The drawing under review shows one solid part. Ordinate dimensions are in mm from its lowest x, y, z. A direction names the side the tool comes from. Coordinates: 2 decimals unless noted, no trailing zeros. Write each loop counter-clockwise with the first axis right and the second up, starting at its lowest first coordinate (ties: lowest second). Pieces come first, ordered by that corner, then holes.
1) Add section D-D, the plane y = 47. State the section outline as (x, z) points.
2) Add section B-B, the plane x = 8. State the section outline as (y, z) points.
3) Mouldability with a two-part tool opening along X and no side actions: class the marked faces 1, 2 and 3 as released by +X, released by -X, zero draft, split by the parting line, or undercut.
4) Add section C-C, the plane z = 4.5. State the section outline as (x, y) points.
5) Machinability: for the marked faces 4, 5 and 6, which of the approach directions +Z, -Z, +X, -X, +Y, -Y give a long, thin tool a straight path to every point of the face, cutting with its end or side? Answer none if there is none.
6) For P1, Ø2, axis at x = 14, z = 3.5, coming from the +Y side; P2, Ø6, axis at x = 20.5, y = 10, coming from the +Z side, all flat-tipped, find the tip position at first contact; note any pin that passes through.
7) Add section A-A, the plane y = 26. State the section outline as (x, z) points.
8) For line 1 (X direction, y = 29, z = 3.5); line 2 (Y direction, x = 8.5, z = 3.5); line 3 (Z direction, x = 21, y = 47.5), list the stretches that pass through material, from the lowest coordinate up.
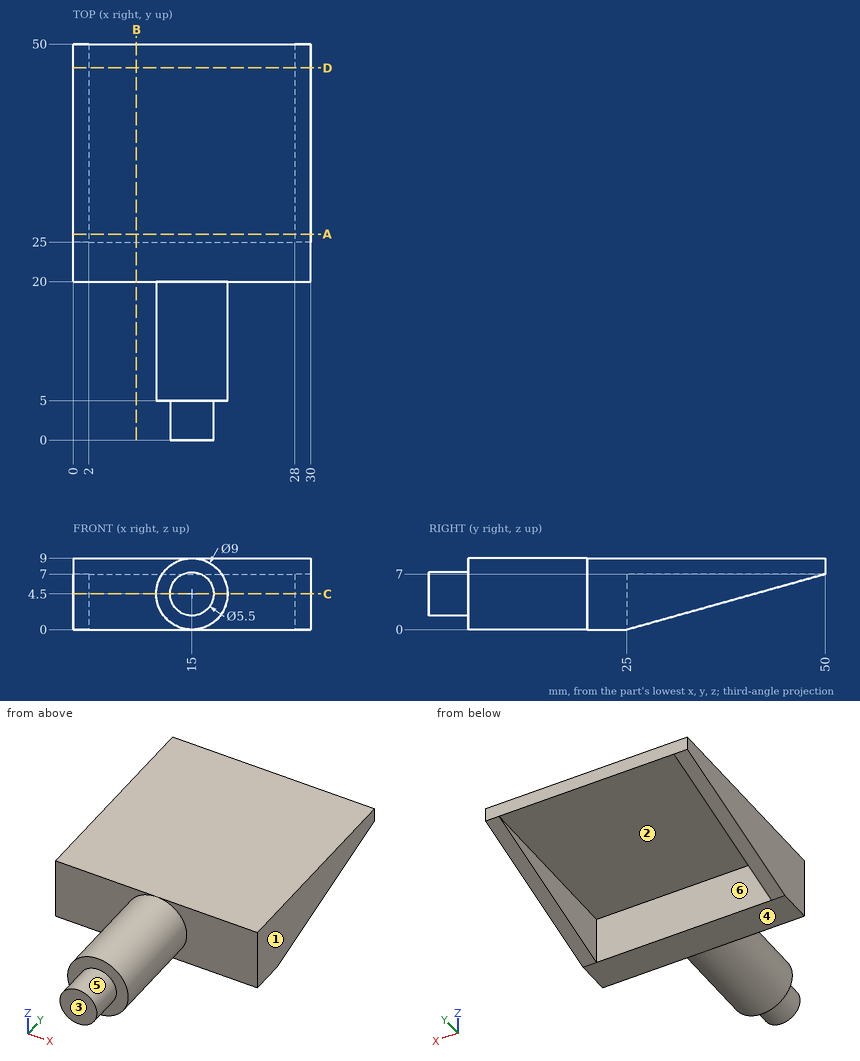
Geometry results:
1. outline: (0, 6.16) - (2, 6.16) - (2, 7) - (28, 7) - (28, 6.16) - (30, 6.16) - (30, 9) - (0, 9) - close
2. outline: (20, 0) - (25, 0) - (25, 7) - (50, 7) - (50, 9) - (20, 9) - close
3. face 1: released by +X
3. face 2: undercut
3. face 3: zero draft
4. outline: (0, 20) - (10.5, 20) - (10.5, 5) - (12.25, 5) - (12.25, 0) - (17.75, 0) - (17.75, 5) - (19.5, 5) - (19.5, 20) - (30, 20) - (30, 41.07) - (28, 41.07) - (28, 25) - (2, 25) - (2, 41.07) - (0, 41.07) - close
5. face 4: -Z, +X, -X, +Y, -Y
5. face 5: -Y
5. face 6: -Z, +Y
6. P1: stops at y = 25
6. P2: stops at z = 8.24
7. outline: (0, 0.28) - (2, 0.28) - (2, 7) - (28, 7) - (28, 0.28) - (30, 0.28) - (30, 9) - (0, 9) - close
8. line 1: x = 0 to 2, 28 to 30
8. line 2: y = 20 to 25
8. line 3: z = 7 to 9
